from build123d import *

# Parameters (mm, degrees)
SKETCH1_W               = 40
SKETCH1_H               = 80
BOSS_EXTRUDE1_DEPTH     = 10
SKETCH2_W               = 30
SKETCH2_H               = 50
BOSS_EXTRUDE2_DEPTH     = 100
SKETCH4_W               = 80
SKETCH4_H               = 30
CUT_EXTRUDE1_DEPTH      = 150
SKETCH3_W               = 30
SKETCH3_H               = 50
SKETCH3_W_2             = 15.3
SKETCH3_H_2             = 30.5
BOSS_EXTRUDE3_DEPTH     = 38
FILLET1_R               = 8
FILLET2_R               = 8
FILLET3_R               = 8
FILLET4_R               = 8
SKETCH5_R               = 1.5
CUT_EXTRUDE2_DEPTH      = 56
CUT_EXTRUDE2_DEPTH_BACK = 26
SKETCH6_R               = 1.5
CUT_EXTRUDE3_DEPTH      = 40


with BuildPart() as part:
    # Sketch1 → Boss-Extrude1 (new body)
    with BuildSketch(Plane.XY):
        with Locations((-7.998819607, 5.424203747)):
            Rectangle(SKETCH1_W, SKETCH1_H)
    extrude(amount=BOSS_EXTRUDE1_DEPTH)

    # Sketch2 → Boss-Extrude2 (add)
    with BuildSketch(Plane(origin=(0, 0, 0), x_dir=(-1, 0, 0), z_dir=(0, 0, -1))):
        with Locations((12.998819607, 5.424203747)):
            Rectangle(SKETCH2_W, SKETCH2_H)
    extrude(amount=BOSS_EXTRUDE2_DEPTH)

    # Sketch4 → Cut-Extrude1 (cut)
    with BuildSketch(Plane.ZY.offset(27.998819607)):
        with Locations((-50, 5.424203747)):
            Rectangle(SKETCH4_W, SKETCH4_H)
    extrude(amount=-CUT_EXTRUDE1_DEPTH, mode=Mode.SUBTRACT)

    # Sketch3 → Boss-Extrude3 (add)
    with BuildSketch(Plane(origin=(0, 0, -100), x_dir=(-1, 0, 0), z_dir=(0, 0, -1))):
        with Locations((12.998819607, 5.424203747)):
            Rectangle(SKETCH3_W, SKETCH3_H)
        with Locations((13.348819607, 5.174203747)):
            Rectangle(SKETCH3_W_2, SKETCH3_H_2, mode=Mode.SUBTRACT)
    extrude(amount=BOSS_EXTRUDE3_DEPTH)

    # Fillet1
    fillet1_edges = [part.edges().sort_by_distance(p)[0] for p in [
        (2.001180393, -19.575796253, -69),
    ]]
    fillet(fillet1_edges, radius=FILLET1_R)

    # Fillet2
    fillet2_edges = [part.edges().sort_by_distance(p)[0] for p in [
        (2.001180393, 30.424203747, -69),
    ]]
    fillet(fillet2_edges, radius=FILLET2_R)

    # Fillet3
    fillet3_edges = [part.edges().sort_by_distance(p)[0] for p in [
        (-27.998819607, -19.575796253, -69),
    ]]
    fillet(fillet3_edges, radius=FILLET3_R)

    # Fillet4
    fillet4_edges = [part.edges().sort_by_distance(p)[0] for p in [
        (-27.998819607, 30.424203747, -69),
    ]]
    fillet(fillet4_edges, radius=FILLET4_R)

    # Sketch5 → Cut-Extrude2 (cut, two sides)
    with BuildSketch(Plane.XZ.offset(-20.424203747)) as cut_extrude2_sk:
        with Locations((-13.348819607, -115)):
            Circle(SKETCH5_R)
        with Locations((-13.348819607, -127)):
            Circle(SKETCH5_R)
    extrude(amount=CUT_EXTRUDE2_DEPTH, mode=Mode.SUBTRACT)
    extrude(cut_extrude2_sk.sketch, amount=-CUT_EXTRUDE2_DEPTH_BACK, mode=Mode.SUBTRACT)

    # Sketch6 → Cut-Extrude3 (cut)
    with BuildSketch(Plane(origin=(0, 0, 0), x_dir=(-1, 0, 0), z_dir=(0, 0, -1))):
        with Locations((20.998819607, 38.424203747)):
            Circle(SKETCH6_R)
        with Locations((-5.001180393, 38.424203747)):
            Circle(SKETCH6_R)
        with Locations((20.998819607, -27.575796253)):
            Circle(SKETCH6_R)
        with Locations((-5.001180393, -27.575796253)):
            Circle(SKETCH6_R)
        with Locations((-7.001180393, 5.424203747)):
            Circle(SKETCH6_R)
    extrude(amount=-CUT_EXTRUDE3_DEPTH, mode=Mode.SUBTRACT)


solid = part.part
The model under review builds one solid part; all positions refer to its coordinate system, in mm. A direction names the side the tool comes from. Round coordinates to 2 decimals unless told otherwise and drop trailing zeros. Loops run counter-clockwise (first coordinate to the right, second up) from the corner with the lowest first, then second, coordinate; pieces in that order, holes last. Notation, with made-up numbers: (38.5, 72.5) -> (46.5, 72.5) arc R25 cw to (46.5, 106.5) -> close; hole circle Ø4 at (68.5, 1). An arc over 180 degrees is marked (long way). One line per question, with ' | ' between items. Start each with the question number.
Item 1: Add section A-A, the plane z = -55.5. Write out the cut boundary in (x, y), then the cut area to 3 significant figures.
Item 2: Add section B-B, the plane x = -8. Write out the cut boundary in (y, z), then the cut area to 3 significant figures.
Item 3: Machinability: for faces 1 (the face through (-13, -19.576, -68)), 2 (the face through (-0.28, 28.02, -68.03)), 3 (the face through (-25.593, -17.295, -69.966)), 4 (the face through (-13, 30.424, -68)), 5 (the face through (-20.999, 5, -119)), which of the approach directions +Z, -Z, +X, -X, +Y, -Y give a long, thin tool a straight path to every point of the face, cutting with its end or side? Answer none if there is none.
Item 4: Add section D-D, the plane z = -96. Write out the cut boundary in (x, y).
Item 5: Add section C-C, the plane y = 19. Write out the cut boundary in (x, z), then the cut area to 3 significant figures.
Item 6: For pin 1 (10 mm diameter, centred on y = 1, z = -96, fed in from +X); pin 2 (4 mm diameter, centred on x = -13.35, z = -115, fed in from -Y); pin 3 (1 mm diameter, centred on x = -2, z = -50, fed in from -Y); pin 4 (2.5 mm diameter, centred on x = -13.35, z = -127, fed in from -Y), all flat-tipped, find the tip position at first contact; note any pin that passes through.
Item 7: Draft analysis for pull direction Z (two halves, no side actions). For faces 6 (the face through (-13, 5, -10)), 7 (the face through (-5.699, 5, -119)), 8 (the face through (5, 6, 0)), state which applies: +Z half, -Z half, draft (parallel to the pull), parting line (faces both ways), or undercut.
Item 8: Wall thickness on line 1 along Z through (x, y) = (-9.5, 17); line 2 along Z through (x, y) = (-5, -9); line 3 along Y through (x, z) = (-12.5, -88.5): over which ranges is each line inside the solid? List them lowest first. Write a range as [from, to].
Return value:
1) outline: (-28, -11.58) arc R8 ccw to (-20, -19.58) -> (-6, -19.58) arc R8 ccw to (2, -11.58) -> (2, -9.58) -> (-28, -9.58) -> close; (-28, 20.42) -> (2, 20.42) -> (2, 22.42) arc R8 ccw to (-6, 30.42) -> (-20, 30.42) arc R8 ccw to (-28, 22.42) -> close | area: 545 mm2
2) outline: (-34.58, 0) -> (-19.58, 0) -> (-19.58, -138) -> (-10.08, -138) -> (-10.08, -100) -> (20.42, -100) -> (20.42, -138) -> (30.42, -138) -> (30.42, 0) -> (45.42, 0) -> (45.42, 10) -> (-34.58, 10) -> close; hole (-9.58, -90) -> (20.42, -90) -> (20.42, -10) -> (-9.58, -10) -> close | area: 4,140 mm2
3) face 1: -Z, +X, -X, -Y | face 2: -Z, +X, +Y | face 3: -Z, -X, -Y | face 4: -Z, +X, -X, +Y | face 5: -Z
4) outline: (-28, -11.58) arc R8 ccw to (-20, -19.58) -> (-6, -19.58) arc R8 ccw to (2, -11.58) -> (2, 22.42) arc R8 ccw to (-6, 30.42) -> (-20, 30.42) arc R8 ccw to (-28, 22.42) -> close
5) outline: (-28, -138) -> (-21, -138) -> (-21, -100) -> (-5.7, -100) -> (-5.7, -138) -> (2, -138) -> (2, -90) -> (-28, -90) -> close; (-28, -10) -> (2, -10) -> (2, 0) -> (12, 0) -> (12, 10) -> (-28, 10) -> close | area: 1,560 mm2
6) pin 1: stops at x = 2 | pin 2: stops at y = -19.58 | pin 3: stops at y = -18.77 | pin 4: passes through
7) face 6: undercut | face 7: draft | face 8: -Z half
8) line 1: z = [-100, -90], [-10, 10] | line 2: z = [-138, -90], [-10, 10] | line 3: y = [-19.58, -9.58], [20.42, 30.42]
